```python
from build123d import *

# Parameters (mm, degrees)
SKETCH1_R           = 97
BOSS_EXTRUDE1_DEPTH = 4
SKETCH2_W           = 60
SKETCH2_H           = 12
CUT_EXTRUDE1_DEPTH  = 10
SKETCH3_W           = 4
SKETCH3_H           = 11
CUT_EXTRUDE2_DEPTH  = 10


with BuildPart() as part:
    # Sketch1 → Boss-Extrude1 (new body)
    with BuildSketch(Plane(origin=(0, 0, 0), x_dir=(1, 0, 0), z_dir=(0, 1, 0))):
        with Locations(Location((0, 0, 0), (0, 0, 270))):  # turned: the seam where the file's is
            Circle(SKETCH1_R)
    extrude(amount=BOSS_EXTRUDE1_DEPTH)

    # Sketch2 → Cut-Extrude1 (cut)
    with BuildSketch(Plane(origin=(0, 4, 0), x_dir=(1, 0, 0), z_dir=(0, 1, 0))):
        with Locations((0, -60)):
            Rectangle(SKETCH2_W, SKETCH2_H)
        with Locations((0, 60)):
            Rectangle(SKETCH2_W, SKETCH2_H)
    extrude(amount=-CUT_EXTRUDE1_DEPTH, mode=Mode.SUBTRACT)

    # Sketch3 → Cut-Extrude2 (cut)
    with BuildSketch(Plane(origin=(0, 4, 0), x_dir=(1, 0, 0), z_dir=(0, 1, 0))):
        with Locations((13.75, -44.75)):
            Rectangle(SKETCH3_W, SKETCH3_H)
        with Locations((13.75, 44.75)):
            Rectangle(SKETCH3_W, SKETCH3_H)
    extrude(amount=-CUT_EXTRUDE2_DEPTH, mode=Mode.SUBTRACT)


solid = part.part
```
Could you check a few things on this model? Use its own coordinates, in mm. Coordinates: 2 decimals unless noted, no trailing zeros. Write each loop counter-clockwise with the first axis right and the second up, starting at its lowest first coordinate (ties: lowest second). Pieces come first, ordered by that corner, then holes. Notation, with made-up numbers: (48.5, 65.25) - (64.5, 65.25) arc R11 cw to (64.5, 86.25) - close; hole circle Ø3 at (45, -28.5). An arc over 180 degrees is marked (long way). Use a Markdown table: item, result.
Q1. Please list where these lines run through material, in increasing order: L1, parallel to Z at x = 28, y = 1.05; L2, parallel to Z at x = -26.5, y = 3.05; L3, parallel to X at y = 2.55, z = 2.
Geometry check:
| item | result |
|---|---|
| L1 | z = -92.87 to -66, -54 to 54, 66 to 92.87 |
| L2 | z = -93.31 to -66, -54 to 54, 66 to 93.31 |
| L3 | x = -96.98 to 96.98 |
Q2. Imagine slicing it at B-B (y = 0.85). List the corners of the cut face in (x, z) for me, and give its area (3 significant figures).
Geometry check:
| item | result |
|---|---|
| outline | circle Ø194 at (0, 0); hole (-30, -66) - (30, -66) - (30, -54) - (-30, -54) - close; hole (-30, 54) - (30, 54) - (30, 66) - (-30, 66) - close; hole (11.75, -50.25) - (15.75, -50.25) - (15.75, -39.25) - (11.75, -39.25) - close; hole (11.75, 39.25) - (15.75, 39.25) - (15.75, 50.25) - (11.75, 50.25) - close |
| area | 28,000 mm2 |
Q3. I'm going to push flat-ended pins straight in: pin 1 Ø2 at (y, z) = (2, 45.5) entering from +X; pin 2 Ø1.2 at (y, z) = (2, 60) entering from +X; pin 3 Ø1 at (y, z) = (2.5, -42.5) entering from +X; pin 4 Ø12 at (x, z) = (26, -19.5) entering from -Y. Where does each tip first touch, or does it pass through?
Geometry check:
| item | result |
|---|---|
| pin 1 | stops at x = 86.19 |
| pin 2 | stops at x = 76.69 |
| pin 3 | stops at x = 87.44 |
| pin 4 | stops at y = 0 |
Q4. Imagine slicing it at C-C (z = -48). List the corners of the cut face in (x, y) for me, and give its area (3 significant figures).
Geometry check:
| item | result |
|---|---|
| outline | (-84.29, 0) - (11.75, 0) - (11.75, 4) - (-84.29, 4) - close; (15.75, 0) - (84.29, 0) - (84.29, 4) - (15.75, 4) - close |
| area | 658 mm2 |
Q5. Imagine slicing it at A-A (x = 0). List the corners of the cut face in (y, z) for me, and give its area (3 significant figures).
Geometry check:
| item | result |
|---|---|
| outline | (0, -97) - (4, -97) - (4, -66) - (0, -66) - close; (0, -54) - (4, -54) - (4, 54) - (0, 54) - close; (0, 66) - (4, 66) - (4, 97) - (0, 97) - close |
| area | 680 mm2 |
Q6. Imagine slicing it at D-D (z = 42.5). List the corners of the cut face in (x, y) for me, and give its area (3 significant figures).
Geometry check:
| item | result |
|---|---|
| outline | (-87.19, 0) - (11.75, 0) - (11.75, 4) - (-87.19, 4) - close; (15.75, 0) - (87.19, 0) - (87.19, 4) - (15.75, 4) - close |
| area | 682 mm2 |
